Verification items for the finished model (mm, model axes). A direction names the side the tool comes from. Round coordinates to 2 decimals unless told otherwise and drop trailing zeros. Loops run counter-clockwise (first coordinate to the right, second up) from the corner with the lowest first, then second, coordinate; pieces in that order, holes last. Notation, with made-up numbers: M 24,63.25 L 38,63.25 A13 ccw 38,76.25 Z; hole C -36,38.25 d9. An arc over 180 degrees is marked long. One line per item, written item: value.
from build123d import *

# Parameters (mm, degrees)
SKETCH_1_W          = 20
SKETCH_1_H          = 20
SKETCH_1_W_2        = 17
SKETCH_1_H_2        = 17
EXTRUDE_1_DEPTH     = 180
SKETCH_2_R          = 2.2
CUT_EXTRUDE_1_DEPTH = 120
SKETCH_3_R          = 2
CUT_EXTRUDE_2_DEPTH = 3
SKETCH_4_R          = 2
CUT_EXTRUDE_3_DEPTH = 20


with BuildPart() as part:
    # 草图1 → 凸台-拉伸1 (new body)
    with BuildSketch(Plane(origin=(0, 0, 0), x_dir=(1, 0, 0), z_dir=(0, 1, 0))):
        Rectangle(SKETCH_1_W, SKETCH_1_H)
        Rectangle(SKETCH_1_W_2, SKETCH_1_H_2, mode=Mode.SUBTRACT)
    extrude(amount=EXTRUDE_1_DEPTH)

    # 草图2 → 切除-拉伸1 (cut)
    with BuildSketch(Plane(origin=(10, 0, 0), x_dir=(0, 0, -1), z_dir=(1, 0, 0))):
        with Locations((0, 135)):
            Circle(SKETCH_2_R)
        with Locations((0, 45)):
            Circle(SKETCH_2_R)
    extrude(amount=-CUT_EXTRUDE_1_DEPTH, mode=Mode.SUBTRACT)

    # 草图3 → 切除-拉伸2 (cut)
    with BuildSketch(Plane.XY.offset(10)):
        with Locations((0, 10)):
            Circle(SKETCH_3_R)
        with Locations((0, 30)):
            Circle(SKETCH_3_R)
        with Locations((0, 50)):
            Circle(SKETCH_3_R)
    extrude(amount=-CUT_EXTRUDE_2_DEPTH, mode=Mode.SUBTRACT)

    # 草图4 → 切除-拉伸3 (cut)
    with BuildSketch(Plane.XY.offset(10)):
        with Locations((0, 74.45)):
            Circle(SKETCH_4_R)
        with Locations((0, 94.45)):
            Circle(SKETCH_4_R)
        with Locations((0, 114.45)):
            Circle(SKETCH_4_R)
    extrude(amount=-CUT_EXTRUDE_3_DEPTH, mode=Mode.SUBTRACT)


solid = part.part
(1) Sectioned sample at B-B on x = -6.25. Enter the section's corners in (y, z), and give its area (3 significant figures).
Completed:
outline: M 0,-10 L 180,-10 L 180,-8.5 L 0,-8.5 Z; M 0,8.5 L 180,8.5 L 180,10 L 0,10 Z
area: 540 mm^2
(2) Thickness scan on L1, parallel to Y at x = 0, z = -8.95; L2, parallel to X at y = 19.5, z = 2. Record the ranges inside material, lowest first. Write a range as from..to.
Completed:
L1: y = 0..72.45, 76.45..92.45, 96.45..112.45, 116.45..180
L2: x = -10..-8.5, 8.5..10
(3) Sectioned sample at A-A on y = 94.45. Enter the section's corners in (x, z), and give its area (3 significant figures).
Completed:
outline: M -10,-10 L -2,-10 L -2,-8.5 L -8.5,-8.5 L -8.5,8.5 L -2,8.5 L -2,10 L -10,10 Z; M 2,-10 L 10,-10 L 10,10 L 2,10 L 2,8.5 L 8.5,8.5 L 8.5,-8.5 L 2,-8.5 Z
area: 99.0 mm^2
(4) Sectioned sample at D-D on y = 55. Enter the section's corners in (x, z).
Completed:
outline: M -10,-10 L 10,-10 L 10,10 L -10,10 Z; hole M -8.5,-8.5 L 8.5,-8.5 L 8.5,8.5 L -8.5,8.5 Z
(5) Tool access check on faces 4 (the face through (-0.26, 76.433, 9.26)), 5 (the face through (8.5, 89, 0)), 6 (the face through (0, 12, 9)). Record the directions out of +Z, -Z, +X, -X, +Y, -Y that give a thin tool (end or side, any length) a straight path to the whole face; none if there is none.
Completed:
face 4: +Z, -Z
face 5: +Y, -Y
face 6: +Z
(6) Sectioned sample at C-C on z = 7. Enter the section's corners in (x, y), and give its area (3 significant figures).
Completed:
outline: M -10,0 L -8.5,0 L -8.5,180 L -10,180 Z; M 8.5,0 L 10,0 L 10,180 L 8.5,180 Z
area: 540 mm^2
(7) Depth check by flat-ended pin: pin 1 Ø4 at (y, z) = (135, 0) entering from -X (3 decimals). Enter the tip coordinate at first touch or a pass-through.
Completed:
pin 1: passes through
(8) Mould release check, pull along Z, two halves, no side actions. Record for faces 1 (the face through (-9, 0, 0)), 2 (the face through (0, 89, -10)), 3 (the face through (0, 89, 8.5)): +Z half, -Z half, draft (parallel to the pull), parting line (faces both ways), or undercut.
Completed:
face 1: draft
face 2: -Z half
face 3: undercut
